The drawing under review shows one solid part. Ordinate dimensions are in mm from its lowest x, y, z. Give positions to 0.01 mm unless a question says otherwise; leave off trailing zeros. Loops run counter-clockwise (first coordinate to the right, second up) from the corner with the lowest first, then second, coordinate; pieces in that order, holes last. Notation, with made-up numbers: M 54.5,20.5 L 113.5,20.5 A20 cw 113.5,35.5 Z; hole C -17.75,29 d7. An arc over 180 degrees is marked long. Put each result on its own line as item: value. Start each with the question number.
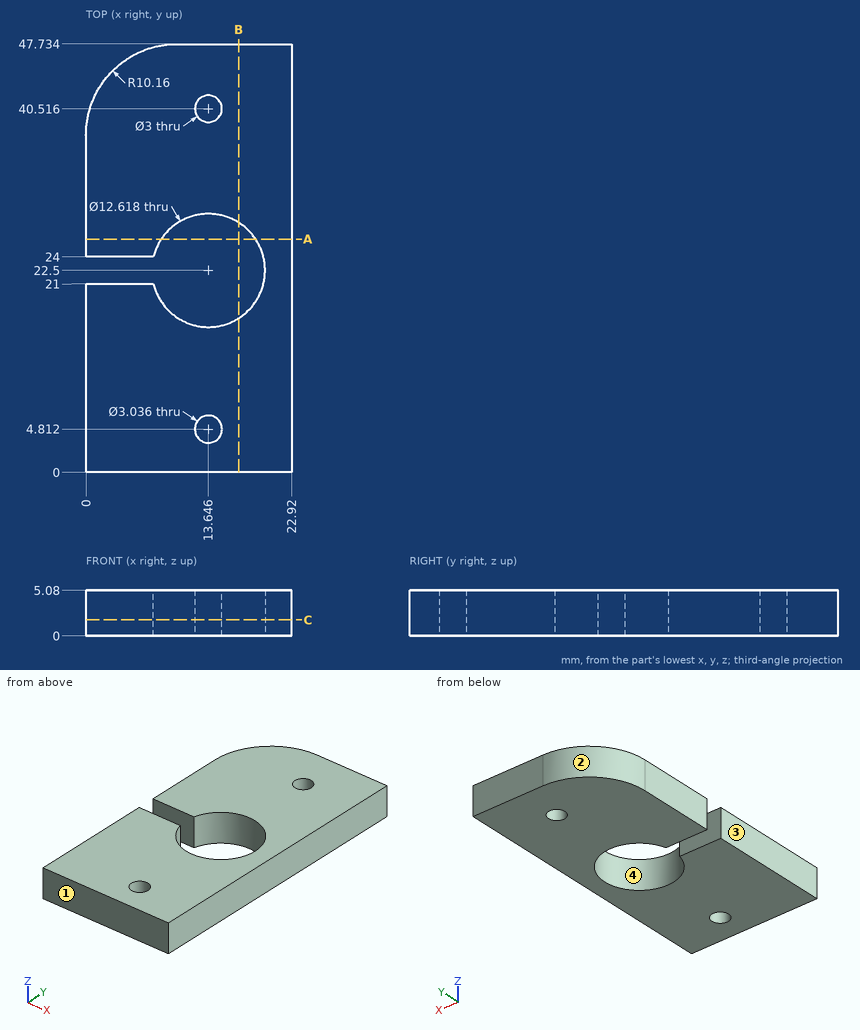
Item 1: Consider section C-C, the plane z = 1.8. Write out the cut boundary in (x, y).
Item 2: To check wall thickness, follow L1, parallel to Y at x = 13, z = 0.95 (1 decimal); L2, parallel to X at y = 18.5, z = 2.35 (1 decimal); L3, parallel to Y at x = 11.25, z = 2.6. State the ranges of each line that lie inside material, in increasing order. Write a range as [from, to].
Item 3: Draft analysis for pull direction Y (two halves, no side actions). For the marked faces 1, 2, 3 and 4, state which applies: +Y half, -Y half, draft (parallel to the pull), parting line (faces both ways), or undercut.
Item 4: Consider section A-A, the plane y = 26. Write out the cut boundary in (x, z) (1 decimal).
Item 5: Consider section B-B, the plane x = 17. Write out the cut boundary in (y, z).
Item 6: Clearance check with flat-ended pins moving along their axes: pin 1 Ø2.5 at (x, y) = (13.65, 40.52) entering from -Z; pin 2 Ø1.5 at (x, z) = (5, 3) entering from +Y. State where each tip first meets the part, or that it passes through.
Report:
1. outline: M 0,0 L 22.92,0 L 22.92,47.73 L 10.16,47.73 A10.16 ccw 0,37.57 L 0,24 L 7.52,24 A6.31 cw long 7.52,21 L 0,21 Z; hole C 13.65,4.81 d3.04; hole C 13.65,40.52 d3
2. L1: [0, 3.4], [6.2, 16.2], [28.8, 39.2], [41.9, 47.7]
2. L2: [0, 8.8], [18.5, 22.9]
2. L3: [0, 16.66], [28.34, 47.73]
3. face 1: -Y half
3. face 2: +Y half
3. face 3: draft
3. face 4: undercut
4. outline: M 0,0 L 8.4,0 L 8.4,5.1 L 0,5.1 Z; M 18.9,0 L 22.9,0 L 22.9,5.1 L 18.9,5.1 Z
5. outline: M 0,0 L 17.16,0 L 17.16,5.08 L 0,5.08 Z; M 27.84,0 L 47.73,0 L 47.73,5.08 L 27.84,5.08 Z
6. pin 1: through
6. pin 2: y = 46.73
